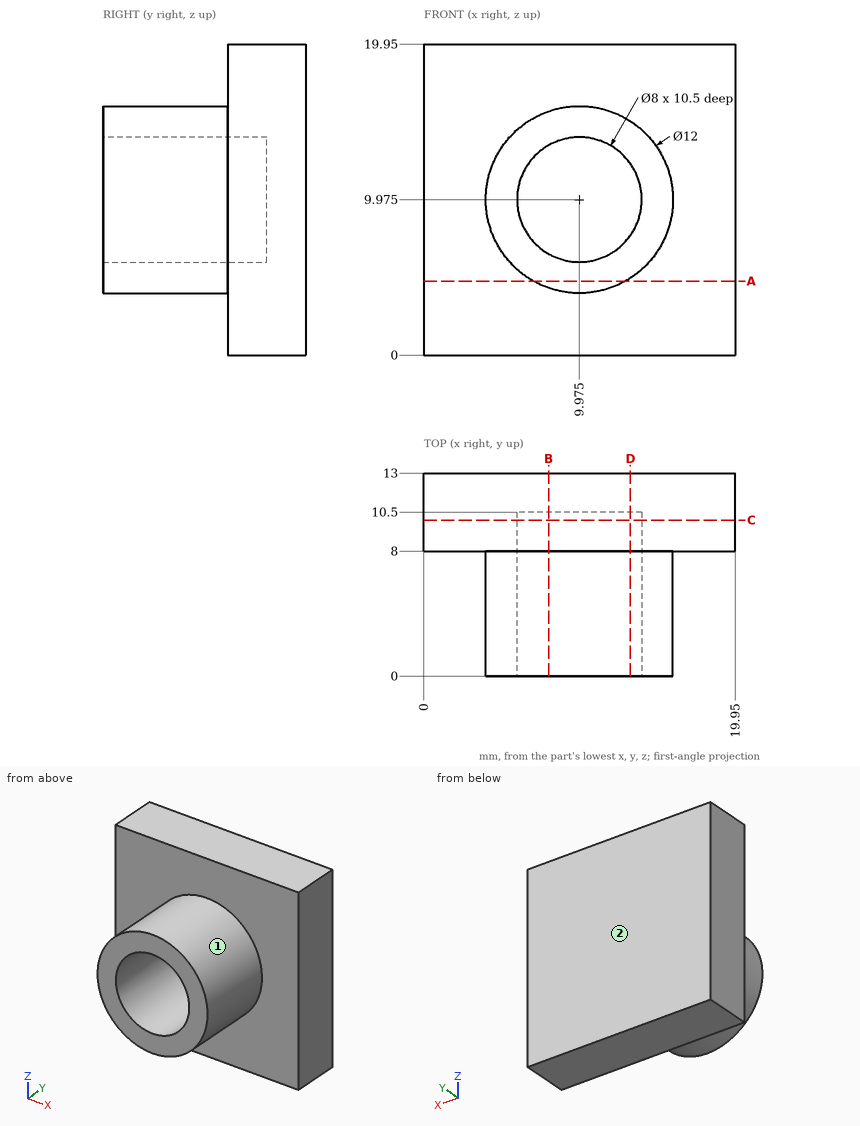
Could you check a few things on this drawing? It's one solid part, dimensions in mm from its lowest x, y, z. A direction names the side the tool comes from. Round coordinates to 2 decimals unless told otherwise and drop trailing zeros. Loops run counter-clockwise (first coordinate to the right, second up) from the corner with the lowest first, then second, coordinate; pieces in that order, holes last. Notation, with made-up numbers: M 7,-12.75 L 20,-12.75 A24 ccw 20,17.25 Z; hole C 81.5,-38.5 d10. An arc over 180 degrees is marked long. Write each question's results on one line, items separated by ' | '. Start each with the question number.
(1) I want a section at C-C (y = 10). Please give me the cut outline in (x, z) (3 decimals).
(2) I want a section at A-A (z = 4.75). Please give me the cut outline in (x, y), then the cut area to 3 significant figures.
(3) If I drill on probe 1 along Y at (x, z) = (11.5, 9.5); probe 2 along Z at (x, y) = (6.75, 7.5); probe 3 along Y at (x, z) = (14.5, 15.75), over which ranges is the centre line in solid material (lowest first)? Write a range as from..to.
(4) I want a section at D-D (x = 13.25). Please give me the cut outline in (y, z), then the cut area to 3 significant figures.
(5) I want a section at B-B (x = 8). Please give me the cut outline in (y, z).
(6) On a 3-axis mill with a long thin cutter (end or side, diameter ignored), from which of +Z, -Z, +X, -X, +Y, -Y can I reach the whole of each face in a straight line? I mean the marked faces 1 and 2. Say none if no direction works.
(7) Will these pins go through, and if not, where does the flat tip stop? P1, Ø2, axis at x = 17.5, z = 4, coming from the -Y side; P2, Ø1.5, axis at y = 2, z = 11.5, coming from the +X side.
Solved:
1) outline: M 0,0 L 19.95,0 L 19.95,19.95 L 0,19.95 Z; hole C 9.975,9.975 d8
2) outline: M 0,8 L 7.03,8 L 7.03,0 L 12.92,0 L 12.92,8 L 19.95,8 L 19.95,13 L 0,13 Z | area: 147 mm²
3) probe 1: y = 10.5..13 | probe 2: z = 4.92..7.61, 12.34..15.03 | probe 3: y = 8..13
4) outline: M 0,4.95 L 8,4.95 L 8,0 L 13,0 L 13,19.95 L 8,19.95 L 8,15 L 0,15 L 0,12.27 L 10.5,12.27 L 10.5,7.68 L 0,7.68 Z | area: 132 mm²
5) outline: M 0,4.31 L 8,4.31 L 8,0 L 13,0 L 13,19.95 L 8,19.95 L 8,15.64 L 0,15.64 L 0,13.45 L 10.5,13.45 L 10.5,6.5 L 0,6.5 Z
6) face 1: -Y | face 2: +Z, -Z, +X, -X, +Y
7) P1: stops at y = 8 | P2: stops at x = 15.92
